Build history of the part. All positions in model axes, mm. Face numbers are marked on the shaded views. A direction names the side the tool comes from. Give positions to 0.01 mm unless a question says otherwise; leave off trailing zeros. Write each loop counter-clockwise with the first axis right and the second up, starting at its lowest first coordinate (ties: lowest second). Pieces come first, ordered by that corner, then holes. Notation, with made-up numbers: M 45.5,74.5 L 56.5,74.5 A9 cw 56.5,84.5 Z; hole C -7,16.5 d1. An arc over 180 degrees is marked long. Return JSON: item names as keys, results as strings. Group by question number.
Q1. Tool access for the marked faces 1, 2 and 3: list every direction of +Z, -Z, +X, -X, +Y, -Y with a clear straight run to the whole face (end or side of a thin tool).
Q2. Band-saw the part on C-C, the plane z = 6.5. Give the cut face in (x, y).
Q3. Wall check: probe 1 along Y at (x, z) = (7.5, 16); probe 2 along Y at (x, z) = (-8, 6.5); probe 3 along Z at (x, y) = (4, 3). Give the ranges that are in metal, low to high.
Q4. Flat gauge pins, fed straight in: pin 1 Ø8 at (x, z) = (10, -11) entering from +Y; pin 2 Ø3 at (x, y) = (-12.5, 45) entering from +Z; pin 3 Ø5 at (x, y) = (0, 59) entering from -Z. Where does each tip first touch, or does it go through?
Q5. Band-saw the part on D-D, the plane x = -6. Give the cut face in (y, z).
Q6. Band-saw the part on B-B, the plane y = 62. Give the cut face in (x, z).
Q7. Band-saw the part on A-A, the plane x = 0. Give the cut face in (y, z).
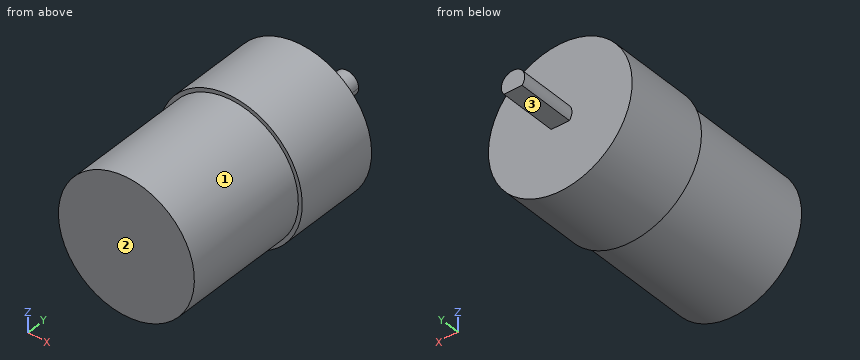
from build123d import *

# Parameters (mm, degrees)
SKETCH_1_R      = 17.5
EXTRUDE_1_DEPTH = 33
SKETCH_2_R      = 18.5
EXTRUDE_2_DEPTH = 22
EXTRUDE_3_DEPTH = 15


with BuildPart() as part:
    # 草图1 → 凸台-拉伸1 (new body)
    with BuildSketch(Plane(origin=(0, 0, 0), x_dir=(1, 0, 0), z_dir=(0, 1, 0))):
        with Locations(Location((0, 0, 0), (0, 0, 270))):
            Circle(SKETCH_1_R)
    extrude(amount=EXTRUDE_1_DEPTH)

    # 草图2 → 凸台-拉伸2 (add)
    with BuildSketch(Plane(origin=(0, 33, 0), x_dir=(1, 0, 0), z_dir=(0, 1, 0))):
        with Locations(Location((0, 0, 0), (0, 0, 270))):
            Circle(SKETCH_2_R)
    extrude(amount=EXTRUDE_2_DEPTH)

    # 草图3 → 凸台-拉伸3 (add)
    with BuildSketch(Plane(origin=(0, 55, 0), x_dir=(1, 0, 0), z_dir=(0, 1, 0))):
        with BuildLine():
            Line((2.339523617, 1.877932173), (0, 1.877932173))
            Line((0, 1.877932173), (-2.339523617, 1.877932173))
            ThreePointArc((-2.339523617, 1.877932173), (-0.99534646, -2.830068095), (3, 0))
            ThreePointArc((3, 0), (2.830068095, 0.99534646), (2.339523617, 1.877932173))
        make_face()
    extrude(amount=EXTRUDE_3_DEPTH)


solid = part.part
From the geometry:
{
 "1": {"face 1": "-Y", "face 2": "+Z, -Z, +X, -X, -Y", "face 3": "-Z, +X, -X, +Y"},
 "2": {"outline": "M -17.32,33 L -16.25,33 L -16.25,0 L 16.25,0 L 16.25,33 L 17.32,33 L 17.32,55 L -17.32,55 Z"},
 "3": {"probe 1": "y = 33 to 55", "probe 2": "y = 0 to 55", "probe 3": "z = -17.04 to 17.04"},
 "4": {"pin 1": "stops at y = 55", "pin 2": "stops at z = 14.87", "pin 3": "stops at z = -1.88"},
 "5": {"outline": "M 0,-16.44 L 33,-16.44 L 33,-17.5 L 55,-17.5 L 55,17.5 L 33,17.5 L 33,16.44 L 0,16.44 Z"},
 "6": {"outline": "M -2.34,-1.88 L 2.34,-1.88 A3 ccw long Z"},
 "7": {"outline": "M 0,-17.5 L 33,-17.5 L 33,-18.5 L 55,-18.5 L 55,-1.88 L 70,-1.88 L 70,3 L 55,3 L 55,18.5 L 33,18.5 L 33,17.5 L 0,17.5 Z"}
}
